Part model, mm, in its own coordinate system. Round coordinates to 2 decimals unless told otherwise and drop trailing zeros. Order: outer loops, then holes, each group sorted by start corner. A loop starts at its lowest first (then second) coordinate and runs counter-clockwise, first axis right, second up. Notation, with made-up numbers: (-30.5, 67.5) -> (-3.5, 67.5) arc R17 ccw to (-3.5, 72.5) -> close; hole circle Ø9 at (-13, 65). An arc over 180 degrees is marked (long way). Return JSON: item names as keys, results as strings. Group by question number.
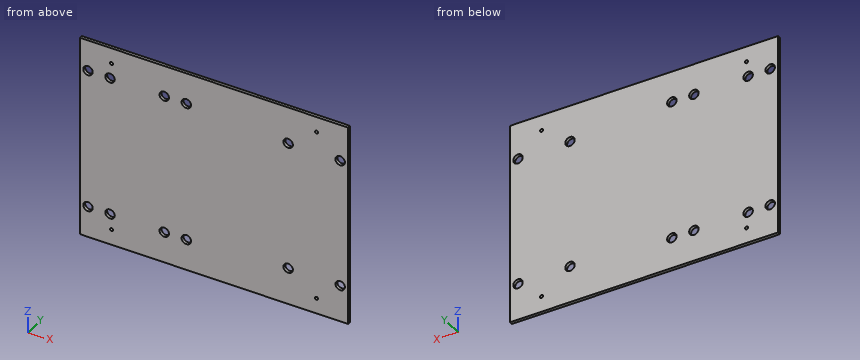
from build123d import *

# Parameters (mm, degrees)
SKETCH1_W           = 170
SKETCH1_H           = 130
SKETCH1_R           = 3
BOSS_EXTRUDE1_DEPTH = 2
SKETCH2_R           = 1
CUT_EXTRUDE1_DEPTH  = 10


with BuildPart() as part:
    # Sketch1 → Boss-Extrude1 (new body)
    with BuildSketch(Plane(origin=(0, 0, 0), x_dir=(1, 0, 0), z_dir=(0, 1, 0))):
        Rectangle(SKETCH1_W, SKETCH1_H)
        with Locations((-80, 45)):
            Circle(SKETCH1_R, mode=Mode.SUBTRACT)
        with Locations((-66, 45)):
            Circle(SKETCH1_R, mode=Mode.SUBTRACT)
        with Locations((-66, -45)):
            Circle(SKETCH1_R, mode=Mode.SUBTRACT)
        with Locations((-80, -45)):
            Circle(SKETCH1_R, mode=Mode.SUBTRACT)
        with Locations((-31.62143128, -45)):
            Circle(SKETCH1_R, mode=Mode.SUBTRACT)
        with Locations((-17.62143128, -45)):
            Circle(SKETCH1_R, mode=Mode.SUBTRACT)
        with Locations((-17.62143128, 45)):
            Circle(SKETCH1_R, mode=Mode.SUBTRACT)
        with Locations((-31.62143128, 45)):
            Circle(SKETCH1_R, mode=Mode.SUBTRACT)
        with Locations((80, 41.33)):
            Circle(SKETCH1_R, mode=Mode.SUBTRACT)
        with Locations((47, 41.33)):
            Circle(SKETCH1_R, mode=Mode.SUBTRACT)
        with Locations((80, -41.33)):
            Circle(SKETCH1_R, mode=Mode.SUBTRACT)
        with Locations((47, -41.33)):
            Circle(SKETCH1_R, mode=Mode.SUBTRACT)
    extrude(amount=BOSS_EXTRUDE1_DEPTH)

    # Sketch2 → Cut-Extrude1 (cut)
    with BuildSketch(Plane(origin=(0, 2, 0), x_dir=(1, 0, 0), z_dir=(0, 1, 0))):
        with Locations((-65, -55)):
            Circle(SKETCH2_R)
        with Locations((-65, 55)):
            Circle(SKETCH2_R)
        with Locations((65, 55)):
            Circle(SKETCH2_R)
        with Locations((65, -55)):
            Circle(SKETCH2_R)
    extrude(amount=-CUT_EXTRUDE1_DEPTH, mode=Mode.SUBTRACT)


solid = part.part
(1) Saw through at B-B, the plane y = 0.65. State how many separate pieces and enclosed holes the cut face has, and give its area (3 significant figures).
(2) Pin check, flat tip, straight feed: P1, Ø9.5, axis at x = 47, z = 41.33, coming from the -Y side. Stop position of the tip, or through.
(3) Saw through at A-A, the plane x = -80. List the corners of the cut face in (y, z), and give its area (3 significant figures).
(4) Probe L1, parallel to Z at x = 80, y = 1.5; L2, parallel to X at y = 0.85, z = -41.33; L3, parallel to Z at x = -80, y = 1.4. List the from-to ranges inside material, lowest first. Write a range as [from, to].
Results are:
{
 "1": {"separate pieces": "1", "enclosed holes": "16", "area": "21,700 mm^2"},
 "2": {"P1": "stops at y = 0"},
 "3": {"outline": "(0, -65) -> (2, -65) -> (2, -48) -> (0, -48) -> close; (0, -42) -> (2, -42) -> (2, 42) -> (0, 42) -> close; (0, 48) -> (2, 48) -> (2, 65) -> (0, 65) -> close", "area": "236 mm^2"},
 "4": {"L1": "z = [-65, -44.33], [-38.33, 38.33], [44.33, 65]", "L2": "x = [-85, 44], [50, 77], [83, 85]", "L3": "z = [-65, -48], [-42, 42], [48, 65]"}
}
